For this review, take the finished solid that the model builds, in its own axes (mm). Face numbers are marked on the shaded views. A direction names the side the tool comes from. Round coordinates to 2 decimals unless told otherwise and drop trailing zeros. Write each loop counter-clockwise with the first axis right and the second up, starting at its lowest first coordinate (ties: lowest second). Pieces come first, ordered by that corner, then holes. Notation, with made-up numbers: M 77,78.25 L 114,78.25 A17 ccw 114,88.25 Z; hole C 36.25,40.25 d5. An arc over 180 degrees is marked long. One line per question, with ' | ' between items.
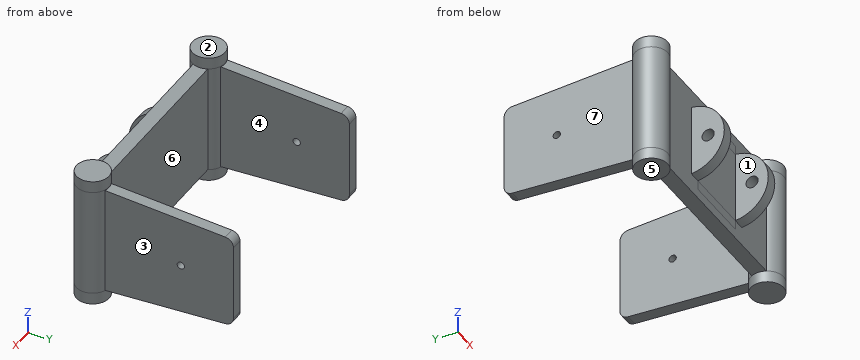
```python
from build123d import *
from build123d.topology import SkipClean

# Parameters (mm, degrees)
SKETCH2_W           = 142.348460158
SKETCH2_H           = 74.966845352
BOSS_EXTRUDE1_DEPTH = 10
SKETCH3_2_R         = 11.189856227
BOSS_EXTRUDE3_DEPTH = 8
SKETCH6_R           = 2.5
BOSS_EXTRUDE5_DEPTH = 4
SKETCH3_R           = 11.189856227
BOSS_EXTRUDE2_DEPTH = 74.966845352
SKETCH4_R           = 11.189856227
BOSS_EXTRUDE4_DEPTH = 8
FILLET1_R           = 6
SKETCH8_R           = 4.167459473
BOSS_EXTRUDE6_DEPTH = 31
CUT_EXTRUDE1_DEPTH  = 31


with BuildPart() as part:
    # Sketch2 → Boss-Extrude1 (new body)
    with BuildSketch(Plane(origin=(0, 0, 0), x_dir=(1, 0, 0), z_dir=(0, 1, 0))):
        Rectangle(SKETCH2_W, SKETCH2_H)
    extrude(amount=BOSS_EXTRUDE1_DEPTH)

    # Sketch3<2> → Boss-Extrude3 (add)
    with BuildSketch(Plane.XY.offset(37.483422676)):
        with Locations(Location((-71.174230079, 5, 0), (0, 0, 333.459309643))):
            Circle(SKETCH3_2_R)
        with Locations(Location((71.174230079, 5, 0), (0, 0, 180))):
            Circle(SKETCH3_2_R)
    extrude(amount=BOSS_EXTRUDE3_DEPTH)

    # Sketch6 → Boss-Extrude5 (add, symmetric)
    with BuildSketch(Plane.ZY.offset(71.174230079)):
        Polygon((31.91575234, 103.68960792), (37.483422676, 10), (37.483422676, 0), (-37.483422676, 0), (-37.483422676, 10), (-31.91575234, 103.68960792), (0, 103.68960792), align=None)
        with Locations((0, 67.56317466)):
            Circle(SKETCH6_R, mode=Mode.SUBTRACT)
    boss_extrude5 = extrude(amount=BOSS_EXTRUDE5_DEPTH, both=True)

    # Sketch3 → Boss-Extrude2 (add)
    with BuildSketch(Plane.XY.offset(37.483422676)):
        with Locations(Location((-71.174230079, 5, 0), (0, 0, 333.459309643))):
            Circle(SKETCH3_R)
        with Locations(Location((71.174230079, 5, 0), (0, 0, 180))):
            Circle(SKETCH3_R)
    extrude(amount=-BOSS_EXTRUDE2_DEPTH)

    # Sketch4 → Boss-Extrude4 (add)
    with SkipClean():  # the faces are left unmerged after this step: merging them gives an invalid solid
        with BuildSketch(Plane(origin=(0, 0, -37.483422676), x_dir=(-1, 0, 0), z_dir=(0, 0, -1))):
            with Locations((-71.174230079, 5)):
                Circle(SKETCH4_R)
            with Locations((71.174230079, 5)):
                Circle(SKETCH4_R)
        extrude(amount=BOSS_EXTRUDE4_DEPTH)

    # Mirror1: Boss-Extrude5 across plane
    add(boss_extrude5.mirror(Plane(origin=(0, 0, 0), x_dir=(0, 0, 1), z_dir=(1, 0, 0))))

    # Fillet1
    fillet1_edges = [part.edges().sort_by_distance(p)[0] for p in [
        (71.174230079, 103.68960792, -31.91575234),
        (-71.174230079, 103.68960792, 31.91575234),
        (-71.174230079, 103.68960792, -31.91575234),
        (71.174230079, 103.68960792, 31.91575234),
    ]]
    fillet(fillet1_edges, radius=FILLET1_R)

    # Sketch8 → Boss-Extrude6 (add, symmetric)
    with BuildSketch(Plane(origin=(0, 0, 0), x_dir=(0, 0, -1), z_dir=(1, 0, 0))):
        with BuildLine():
            Line((-24.669316097, 0), (0, 0))
            Line((0, 0), (24.669316097, 0))
            ThreePointArc((24.669316097, 0), (0, -22.602874457), (-24.669316097, 0))
        make_face()
        with Locations((0, -11.517091371)):
            Circle(SKETCH8_R, mode=Mode.SUBTRACT)
    extrude(amount=BOSS_EXTRUDE6_DEPTH, both=True)

    # Sketch9 → Cut-Extrude1 (cut, symmetric)
    with BuildSketch(Plane.XY):
        Polygon((0, 0), (-23, 0), (-23, -24.601759038), (-2.110664843, -24.601759038), (23, -24.601759038), (23, 0), align=None)
    extrude(amount=CUT_EXTRUDE1_DEPTH, both=True, mode=Mode.SUBTRACT)


solid = part.part
```
Item 1: Take a section at D-D (y = 5). Write out the cut boundary in (x, z), then the cut area to 3 significant figures.
Results:
outline: M -82.36,-45.48 L -59.98,-45.48 L -59.98,-37.48 L 59.98,-37.48 L 59.98,-45.48 L 82.36,-45.48 L 82.36,45.48 L 59.98,45.48 L 59.98,37.48 L -59.98,37.48 L -59.98,45.48 L -82.36,45.48 Z | area: 13,100 mm2
Item 2: Take a section at A-A (y = 53). Write out the cut boundary in (x, z), then the cut area to 3 significant figures.
Results:
outline: M -75.17,-34.93 L -67.17,-34.93 L -67.17,34.93 L -75.17,34.93 Z; M 67.17,-34.93 L 75.17,-34.93 L 75.17,34.93 L 67.17,34.93 Z | area: 1,120 mm2
Item 3: Machinability: for the marked faces 1, 2, 3 and 4, which of the approach directions +Z, -Z, +X, -X, +Y, -Y give a long, thin tool a straight path to every point of the face, cutting with its end or side? Answer none if there is none.
Results:
face 1: +Z, -Z, -Y | face 2: +Z, +X, -X, +Y, -Y | face 3: +Z, -Z, +X, +Y | face 4: +Z, -Z, +Y
Item 4: Mouldability with a two-part tool opening along X and no side actions: class the marked faces 5, 6 and 7 as +X half, -X half, draft (parallel to the pull), parting line (faces both ways), or undercut.
Results:
face 5: draft | face 6: undercut | face 7: -X half
Item 5: Take a section at B-B (x = -72). Write out the cut boundary in (y, z), then the cut area to 3 significant figures.
Results:
outline: M -6.16,-45.48 L 16.16,-45.48 L 16.16,-37.12 L 98.05,-32.25 A6 ccw 103.69,-26.26 L 103.69,26.26 A6 ccw 98.05,32.25 L 16.16,37.12 L 16.16,45.48 L -6.16,45.48 Z; hole C 67.56,0 d5 | area: 8,040 mm2
Item 6: Insertion check: pin 1 Ø3 at (y, z) = (43, -15) entering from +X; pin 2 Ø10 at (x, y) = (-32.5, 19.5) entering from -Z; pin 3 Ø1.5 at (x, z) = (27.5, -31) entering from -Y; pin 4 Ø13.5 at (y, z) = (-11.52, 0) entering from +X. Each pin has a flat end and moves straight along its axis. Give the tip position at first contact, or say it passes through.
Results:
pin 1: x = 75.17 | pin 2: through | pin 3: y = 0 | pin 4: x = 76.63
Item 7: To check wall thickness, follow line 1 along X through (y, z) = (54, 17); line 2 along Y through (x, z) = (28, 0); line 3 along Y through (x, z) = (-0.5, 36.5). State the ranges of each line that lie inside material, in increasing order. Write a range as from..to.
Results:
line 1: -75.17..-67.17, 67.17..75.17 | line 2: -22.6..-15.68, -7.35..10 | line 3: 0..10
Item 8: Take a section at C-C (z = 0). State how many separate pieces and enclosed holes the cut face has, then the cut area to 3 significant figures.
Results:
separate pieces: 5 | enclosed holes: 0 | area: 3,550 mm2
